Build history of the part. All positions in model axes, mm. Face numbers are marked on the shaded views. A direction names the side the tool comes from. Round coordinates to 2 decimals unless told otherwise and drop trailing zeros. Loops run counter-clockwise (first coordinate to the right, second up) from the corner with the lowest first, then second, coordinate; pieces in that order, holes last. Notation, with made-up numbers: (26, 17) - (52, 17) arc R16 cw to (52, 33) - close; hole circle Ø3 at (65, 81). An arc over 180 degrees is marked (long way). Put each result on its own line as item: value. Start each with the question number.
from build123d import *

# Parameters (mm, degrees)
SKETCH064_R     = 4.5
PAD029_DEPTH    = 1.4
SKETCH065_R     = 4.5
PAD030_DEPTH    = 5.7
SKETCH066_R     = 3.325
POCKET031_DEPTH = 5.7
FILLET002_R     = 0.8


with BuildPart() as part:
    # Sketch064 → Pad029 (new body)
    with BuildSketch(Plane.XY):
        with Locations((-7.58, -28.79)):
            Circle(SKETCH064_R)
    extrude(amount=-PAD029_DEPTH)

    # Sketch065 → Pad030 (join)
    with BuildSketch(Plane.XY):
        with Locations((-7.58, -28.79)):
            Circle(SKETCH065_R)
    extrude(amount=PAD030_DEPTH)

    # Sketch066 → Pocket031 (cut)
    with BuildSketch(Plane.XY):
        with Locations((-7.58, -28.79)):
            Circle(SKETCH066_R)
    extrude(amount=POCKET031_DEPTH, mode=Mode.SUBTRACT)

    # Fillet002
    fillet002_edges = [part.edges().sort_by_distance(p)[0] for p in [
        (-10.905, -28.79, 5.7),
    ]]
    fillet(fillet002_edges, radius=FILLET002_R)


with BuildPart() as part_1:
    # Body009 placement: moved
    add(part.part.moved(Location((0, 0, 16.4))))


solid = part_1.part
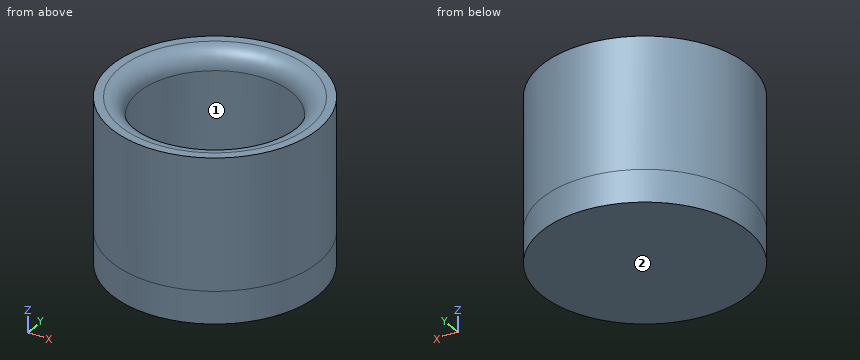
1) Slice it at D-D, the plane z = 21.5. Write the cut outline in (x, y).
2) Slice it at A-A, the plane y = -28.79. Write the cut outline in (x, z) (3 decimals), and give its area (3 significant figures).
3) Slice it at B-B, the plane x = -7.58. Write the cut outline in (y, z) (3 decimals).
4) Drill centre lines: line 1 (Y direction, x = -7.5, z = 19.75); line 2 (Z direction, x = -7.5, y = -27); line 3 (X direction, y = -27.5, z = 19.5). Where is each one in solid material? Low to high. Write a range as [from, to].
5) Which spindle directions (+Z, -Z, +X, -X, +Y, -Y) get a long thin tool onto all of the face, cutting with end or side? Do the marked faces 1 and 2. Say none if no direction does.
6) Slice it at C-C, the plane z = 17.5. Write the cut outline in (x, y) (3 decimals), and give its area (3 significant figures).
7) Drop flat-ended pins along their axis: pin 1 Ø2 at (x, z) = (-10.5, 17) entering from -Y; pin 2 Ø1.5 at (y, z) = (-31, 17.5) entering from +X. Give the stop position or say it passes through.
Taken from the geometry:
1. outline: circle Ø9 at (-7.58, -28.79); hole circle Ø6.7 at (-7.58, -28.79)
2. outline: (-12.08, 15) - (-3.08, 15) - (-3.08, 22.1) - (-3.455, 22.1) arc R0.8 ccw to (-4.255, 21.3) - (-4.255, 16.4) - (-10.905, 16.4) - (-10.905, 21.3) arc R0.8 ccw to (-11.705, 22.1) - (-12.08, 22.1) - close
2. area: 25.7 mm2
3. outline: (-33.29, 15) - (-24.29, 15) - (-24.29, 22.1) - (-24.665, 22.1) arc R0.8 ccw to (-25.465, 21.3) - (-25.465, 16.4) - (-32.115, 16.4) - (-32.115, 21.3) arc R0.8 ccw to (-32.915, 22.1) - (-33.29, 22.1) - close
4. line 1: y = [-33.29, -32.11], [-25.47, -24.29]
4. line 2: z = [15, 16.4]
4. line 3: x = [-11.89, -10.64], [-4.52, -3.27]
5. face 1: +Z
5. face 2: -Z, +X, -X, +Y, -Y
6. outline: circle Ø9 at (-7.58, -28.79); hole circle Ø6.65 at (-7.58, -28.79)
6. area: 28.9 mm2
7. pin 1: stops at y = -32.86
7. pin 2: stops at x = -3.32
